Model file for the job. Use its own axes, mm. A direction names the side the tool comes from. Give positions to 0.01 mm unless a question says otherwise; leave off trailing zeros. Write each loop counter-clockwise with the first axis right and the second up, starting at its lowest first coordinate (ties: lowest second). Pieces come first, ordered by that corner, then holes.
```python
from build123d import *

# Parameters (mm, degrees)
SKETCH1_R           = 15.24
BOSS_EXTRUDE1_DEPTH = 5.08
BOSS_EXTRUDE3_DEPTH = 2.54
CIRPATTERN1_COUNT   = 48
SKETCH6_R           = 4.064
CUT_EXTRUDE1_DEPTH  = 2.54
SKETCH7_R           = 2.000000064
CUT_EXTRUDE2_DEPTH  = 2.54


with BuildPart() as part:
    # Sketch1 → Boss-Extrude1 (new body)
    with BuildSketch(Plane(origin=(0, 0, 0), x_dir=(1, 0, 0), z_dir=(0, 1, 0))):
        with Locations(Location((0, 0, 0), (0, 0, 270))):
            Circle(SKETCH1_R)
    extrude(amount=BOSS_EXTRUDE1_DEPTH)

    # Sketch3 → Boss-Extrude3 (add)
    with BuildSketch(Plane(origin=(0, 5.08, 0), x_dir=(1, 0, 0), z_dir=(0, 1, 0))):
        Polygon((0, 21.59), (3.969953129, 14.713839477), (-3.969953129, 14.713839477), align=None)
    boss_extrude3 = extrude(amount=-BOSS_EXTRUDE3_DEPTH)

    # CirPattern1: Boss-Extrude3 ×48 about axis
    cirpattern1_axis = Axis((0, 0, 0), (0, 1, 0))
    for i in range(1, CIRPATTERN1_COUNT):
        add(boss_extrude3.rotate(cirpattern1_axis, i * 360 / CIRPATTERN1_COUNT))

    # Sketch6 → Cut-Extrude1 (cut)
    with BuildSketch(Plane.XZ):
        with Locations(Location((0, 0, 0), (0, 0, 270))):
            Circle(SKETCH6_R)
    extrude(amount=-CUT_EXTRUDE1_DEPTH, mode=Mode.SUBTRACT)

    # Sketch7 → Cut-Extrude2 (cut)
    with BuildSketch(Plane(origin=(0, 5.08, 0), x_dir=(1, 0, 0), z_dir=(0, 1, 0))):
        with Locations(Location((0, 0, 0), (0, 0, 270))):
            Circle(SKETCH7_R)
    extrude(amount=-CUT_EXTRUDE2_DEPTH, mode=Mode.SUBTRACT)


solid = part.part
```
1. Slice it at B-B, the plane x = 12. Write the cut outline in (y, z).
Calculated:
outline: (0, -9.39) - (2.54, -9.39) - (2.54, -16.65) - (5.08, -16.65) - (5.08, 16.65) - (2.54, 16.65) - (2.54, 9.39) - (0, 9.39) - close
2. Probe probe 1 along Z at (x, y) = (17, 3.1) (3 decimals); probe 2 along Y at (x, z) = (0, -2.5); probe 3 along Z at (x, y) = (14, 3.1). List the from-to ranges inside material, lowest first.
Calculated:
probe 1: z = -13.126 to -12.833, -10.795 to 10.795, 12.833 to 13.126
probe 2: y = 2.54 to 5.08
probe 3: z = -14.93 to 14.93
3. Slice it at A-A, the plane y = 1.15. Write the cut outline in (x, z), and give its area (3 significant figures).
Calculated:
outline: circle Ø30.48 at (0, 0); hole circle Ø8.13 at (0, 0)
area: 678 mm2
4. Which spindle directions (+Z, -Z, +X, -X, +Y, -Y) get a long thin tool onto all of the face, cutting with end or side? Do faces 1 (the flat face through (-20.248, 3.828, -3.298)), 2 (the flat face through (20.474, 3.828, -0.644)), 3 (the flat face through (-11.99, 3.83, -16.65)), 4 (the flat face through (11.99, 3.83, 16.65)), 5 (the flat face through (-1, 2.54, 2)). Say none if no direction does.
Calculated:
face 1: -X, +Y, -Y
face 2: +X, +Y, -Y
face 3: -Z, +Y, -Y
face 4: +Z, +Y, -Y
face 5: -Y
5. Pull direction Z, two halves, no side cores. Call faces 6 (the flat face through (-0.63, 3.83, 20.5)), 7 (the flat face through (-19.943, 3.828, -4.677)), 8 (the flat face through (-16.635, 3.828, -11.953)), 9 (the flat face through (-3.311, 3.828, -20.215)): +Z half, -Z half, draft (parallel to the pull), parting line (faces both ways), or undercut.
Calculated:
face 6: +Z half
face 7: undercut
face 8: undercut
face 9: -Z half
6. Slice it at C-C, the plane z = 10. Write the cut outline in (x, y), and give its area (3 significant figures).
Calculated:
outline: (-18.24, 2.54) - (-11.5, 2.54) - (-11.5, 0) - (11.5, 0) - (11.5, 2.54) - (18.24, 2.54) - (18.24, 5.08) - (-18.24, 5.08) - close
area: 151 mm2
7. Pin check, flat tips, straight feed: P1, Ø3, axis at x = 17.5, y = 3.5, coming from the -Z side; P2, Ø3, axis at x = -17.5, y = 4, coming from the +Z side; P3, Ø1.3, axis at y = 3.5, z = -17.5, coming from the +X side. Stop position of each tip, or through.
Calculated:
P1: stops at z = -13.14
P2: stops at z = 13.14
P3: stops at x = 13.14
